```python
from build123d import *

# Parameters (mm, degrees)
F0_R     = 17.45
F0_R_2   = 13.6
F1_DEPTH = 250
F2_R     = 2
F4_R     = 2


# Not quite as in the source:
# - a fillet or chamfer that OpenCascade refuses, or shapes differently, is made with other operations: its cross-section is extruded or revolved along the edge and cut away or added


with BuildPart() as f1:
    # F0 (on Top) → F1 (new body)
    with BuildSketch(Plane.XY):
        Circle(F0_R)
        Circle(F0_R_2, mode=Mode.SUBTRACT)
    extrude(amount=F1_DEPTH)

    # F2
    f2_edges = [f1.edges().sort_by_distance(p)[0] for p in [
        (-13.6, 0, 250),
    ]]
    fillet(f2_edges, radius=F2_R)

    # F3: fillet of radius 2 on 1 edges, made by hand

    # F3_s1 → F3_t2 (revolve, cut)
    with BuildSketch(Plane.XZ):
        with BuildLine():
            ThreePointArc((15.6, 250), (16.9162878299, 249.3657799834), (17.45, 248.0056329325))
            Line((17.45, 248.0056329325), (17.45, 250))
            Line((17.45, 250), (15.6, 250))
        make_face()
    revolve(axis=Axis((0, 0, 250), (0, 0, 1)), mode=Mode.SUBTRACT)

    # F4
    f4_edges = [f1.edges().sort_by_distance(p)[0] for p in [
        (-13.6, 0, 0),
    ]]
    fillet(f4_edges, radius=F4_R)

    # F5: fillet of radius 2 on 1 edges, made by hand

    # F5_s1 → F5_t2 (revolve, cut)
    with BuildSketch(Plane.XZ):
        with BuildLine():
            ThreePointArc((15.6, 0), (16.9162878299, 0.6342200166), (17.45, 1.9943670675))
            Line((17.45, 1.9943670675), (17.45, 0))
            Line((17.45, 0), (15.6, 0))
        make_face()
    revolve(axis=Axis((0, 0, 0), (0, 0, 1)), mode=Mode.SUBTRACT)


solid = f1.part
```
Check sheet for the modelled part. Datum: model origin and axes. Units: mm. Round coordinates to 2 decimals unless told otherwise and drop trailing zeros. Order: outer loops, then holes, each group sorted by start corner. A loop starts at its lowest first (then second) coordinate and runs counter-clockwise, first axis right, second up. Notation, with made-up numbers: M 34,83 L 85,83 A20 ccw 85,122 Z; hole C 77.5,14.25 d11. An arc over 180 degrees is marked long. Answer in a Markdown table with one row per item.
(1) Section check A-A on x = 0. Record the boundary of the cut face in (y, z), plus the area to 3 significant figures.
Findings:
| item | result |
|---|---|
| outline | M -17.45,1.99 A2 ccw -15.6,0 A2 ccw -13.6,2 L -13.6,248 A2 ccw -15.6,250 A2 ccw -17.45,248.01 Z; M 13.6,2 A2 ccw 15.6,0 A2 ccw 17.45,1.99 L 17.45,248.01 A2 ccw 15.6,250 A2 ccw 13.6,248 Z |
| area | 1,920 mm^2 |
(2) Gauge pin test, flat ends, axial feed: pin 1 (2 mm diameter, centred on x = 3, z = 174.5, fed in from +Y) (3 decimals); pin 2 (6 mm diameter, centred on y = -11.5, z = 71, fed in from -X); pin 3 (5 mm diameter, centred on x = 7, z = 55, fed in from +Y); pin 4 (4 mm diameter, centred on x = 9.5, y = 4, fed in from +Z). Record the tip position at first contact, or that the pin passes through.
Findings:
| item | result |
|---|---|
| pin 1 | stops at y = 17.335 |
| pin 2 | stops at x = -15.24 |
| pin 3 | stops at y = 16.86 |
| pin 4 | passes through |
(3) Draft check along Y on faces 1 (the cylindrical face through (-3.783, -17.035, 123.278)), 2 (the cylindrical face through (-2.948, -13.277, 123.278)). Enter one of: +Y half, -Y half, draft (parallel to the pull), parting line (faces both ways), or undercut.
Findings:
| item | result |
|---|---|
| face 1 | parting line |
| face 2 | undercut |
(4) Material ranges on line 1 along Y through (x, z) = (0, 124); line 2 along Y through (x, z) = (11, 67); line 3 along X through (y, z) = (4.5, 39), recorded low to high. Write a range as from..to.
Findings:
| item | result |
|---|---|
| line 1 | y = -17.45..-13.6, 13.6..17.45 |
| line 2 | y = -13.55..-8, 8..13.55 |
| line 3 | x = -16.86..-12.83, 12.83..16.86 |
(5) Section check C-C on z = 43. Record the boundary of the cut face in (x, y).
Findings:
| item | result |
|---|---|
| outline | C 0,0 d34.9; hole C 0,0 d27.2 |
